Answer from the drawing. Dimensions are ordinates in mm from the lowest x, y and z of the part. Round coordinates to 2 decimals unless told otherwise and drop trailing zeros. Loops run counter-clockwise (first coordinate to the right, second up) from the corner with the lowest first, then second, coordinate; pieces in that order, holes last. Notation, with made-up numbers: (77.5, 53.5) - (122.5, 53.5) arc R19 ccw to (122.5, 58.5) - close; hole circle Ø5 at (80.5, 53.25). An arc over 180 degrees is marked (long way). One line per question, with ' | ' between items. Start each with the question number.
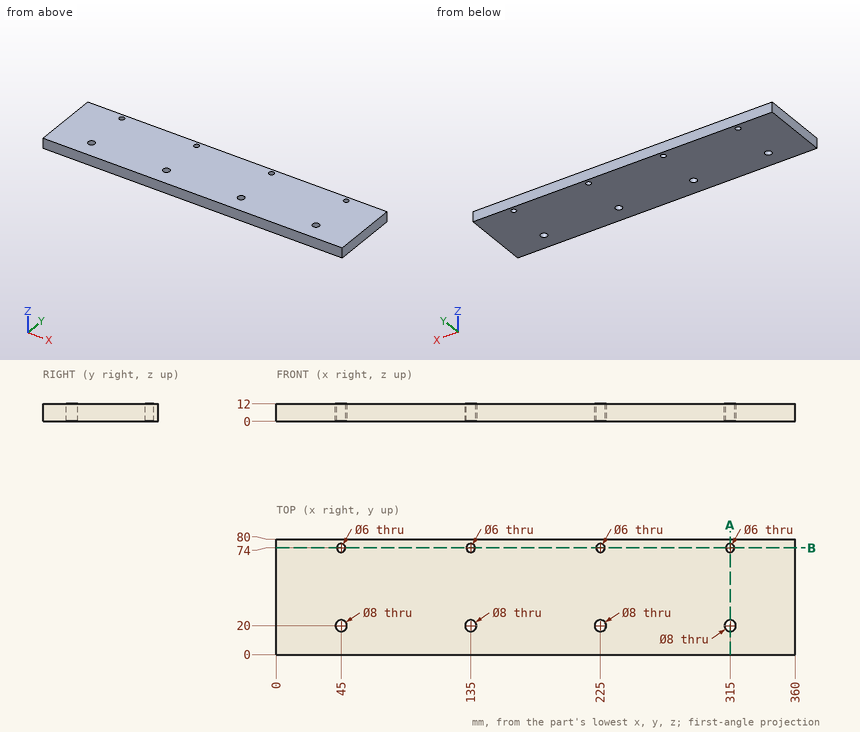
(1) Find section A-A on x = 315. Write down the section's boundary in (y, z), plus the area to 3 significant figures.
(2) Find section B-B on y = 74. Write down the section's boundary in (x, z).
(3) Consider L1, parallel to Y at x = 225, z = 8.5; L2, parallel to X at y = 76, z = 7.25. Determine where each line is inside the solid, lowest interval first.
Answer below:
1) outline: (0, 0) - (16, 0) - (16, 12) - (0, 12) - close; (24, 0) - (71, 0) - (71, 12) - (24, 12) - close; (77, 0) - (80, 0) - (80, 12) - (77, 12) - close | area: 792 mm2
2) outline: (0, 0) - (42, 0) - (42, 12) - (0, 12) - close; (48, 0) - (132, 0) - (132, 12) - (48, 12) - close; (138, 0) - (222, 0) - (222, 12) - (138, 12) - close; (228, 0) - (312, 0) - (312, 12) - (228, 12) - close; (318, 0) - (360, 0) - (360, 12) - (318, 12) - close
3) L1: 0 to 16, 24 to 71, 77 to 80 | L2: 0 to 42.76, 47.24 to 132.76, 137.24 to 222.76, 227.24 to 312.76, 317.24 to 360
